Check sheet for the modelled part. Datum: model origin and axes. Units: mm. Face numbers are marked on the shaded views. A direction names the side the tool comes from. Coordinates: 2 decimals unless noted, no trailing zeros. Loops run counter-clockwise (first coordinate to the right, second up) from the corner with the lowest first, then second, coordinate; pieces in that order, holes last. Notation, with made-up numbers: M 35,24 L 76,24 A4 ccw 76,29 Z; hole C 50.25,78.5 d7. An arc over 180 degrees is marked long. Answer in a Markdown table with one row per item. Add a question column.
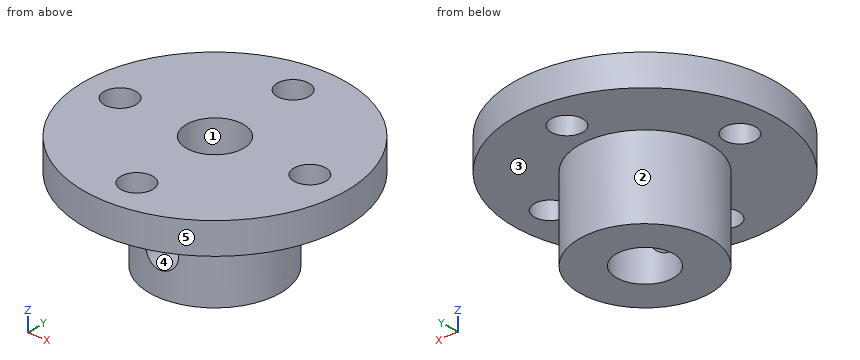
```python
from build123d import *

# Parameters (mm, degrees)
SKETCH1_R           = 8
SKETCH1_R_2         = 3.5
BOSS_EXTRUDE1_DEPTH = 10
SKETCH2_R           = 16
SKETCH2_R_2         = 3.5
BOSS_EXTRUDE2_DEPTH = 3.81
SKETCH3_R           = 1.95
CUT_EXTRUDE1_DEPTH  = 27.508792881
SKETCH4_R           = 2
CUT_EXTRUDE2_DEPTH  = 27.508792881


with BuildPart() as part:
    # Sketch1 → Boss-Extrude1 (new body)
    with BuildSketch(Plane.XY):
        Circle(SKETCH1_R)
        Circle(SKETCH1_R_2, mode=Mode.SUBTRACT)
    extrude(amount=BOSS_EXTRUDE1_DEPTH)

    # Sketch2 → Boss-Extrude2 (add)
    with BuildSketch(Plane.XY.offset(10)):
        with Locations(Location((0, 0, 0), (0, 0, 180))):
            Circle(SKETCH2_R)
        Circle(SKETCH2_R_2, mode=Mode.SUBTRACT)
    extrude(amount=BOSS_EXTRUDE2_DEPTH)

    # Sketch3 → Cut-Extrude1 (cut, through all)
    with BuildSketch(Plane.XY.offset(13.81)):
        with Locations((0, 11.43)):
            Circle(SKETCH3_R)
        with Locations((11.43, 0)):
            Circle(SKETCH3_R)
        with Locations((0, -11.43)):
            Circle(SKETCH3_R)
        with Locations((-11.43, 0)):
            Circle(SKETCH3_R)
    extrude(amount=-CUT_EXTRUDE1_DEPTH, mode=Mode.SUBTRACT)

    # Sketch4 → Cut-Extrude2 (cut, through all)
    with BuildSketch(Plane(origin=(0, 0, 0), x_dir=(1, 0, 0), z_dir=(0, 1, 0))):
        with Locations(Location((0, -5, 0), (0, 0, 270))):
            Circle(SKETCH4_R)
    extrude(amount=-CUT_EXTRUDE2_DEPTH, mode=Mode.SUBTRACT)


solid = part.part
```
Q1. Access from +Z, -Z, +X, -X, +Y, -Y to the whole of each face (thin tool, end or side, straight path). Record for the marked faces 1 and 2.
Q2. Thickness scan on L1, parallel to Y at x = 0, z = 11.25; L2, parallel to Y at x = 0, z = 8; L3, parallel to X at y = -4.5, z = 4.25. Record the ranges inside material, lowest first.
Q3. Cross-section at A-A (x = 0). Record the cut outline in (y, z).
Q4. Cross-section at B-B (y = -1). Record the cut outline in (x, z).
Q5. Cross-section at C-C (x = 11.43). Record the cut outline in (y, z), plus the area to 3 significant figures.
Q6. Cross-section at D-D (z = 13). Record the cut outline in (x, y), plus the area to 3 significant figures.
Q7. Mould release check, pull along X, two halves, no side actions. Record for the marked faces 3, 4 and 5: released by +X, released by -X, zero draft, split by the parting line, or undercut.
Q8. Go/stop test with flat-tipped pins: pin 1 (1.5 mm diameter, centred on y = -6.5, z = 10, fed in from +X); pin 2 (6 mm diameter, centred on x = 0, y = -11.43, fed in from -Z); pin 3 (2 mm diameter, centred on y = -5.5, z = 3, fed in from +X); pin 4 (3 mm diameter, centred on x = 0, y = 11.43, fed in from +Z). Record where each tip stops, or that it passes through.
Answer key:
| question | item | result |
|---|---|---|
| 1 | face 1 | +Z, -Z |
| 1 | face 2 | -Z |
| 2 | L1 | -16 to -13.38, -9.48 to -3.5, 3.5 to 9.48, 13.38 to 16 |
| 2 | L2 | -8 to -3.5, 3.5 to 8 |
| 2 | L3 | -6.61 to -1.85, 1.85 to 6.61 |
| 3 | outline | M -16,10 L -13.38,10 L -13.38,13.81 L -16,13.81 Z; M -9.48,10 L -8,10 L -8,7 L -3.5,7 L -3.5,13.81 L -9.48,13.81 Z; M -8,0 L -3.5,0 L -3.5,3 L -8,3 Z; M 3.5,0 L 8,0 L 8,10 L 9.48,10 L 9.48,13.81 L 3.5,13.81 Z; M 13.38,10 L 16,10 L 16,13.81 L 13.38,13.81 Z |
| 4 | outline | M -15.97,10 L -13.1,10 L -13.1,13.81 L -15.97,13.81 Z; M -9.76,10 L -7.94,10 L -7.94,0 L -3.35,0 L -3.35,13.81 L -9.76,13.81 Z; M 3.35,0 L 7.94,0 L 7.94,10 L 9.76,10 L 9.76,13.81 L 3.35,13.81 Z; M 13.1,10 L 15.97,10 L 15.97,13.81 L 13.1,13.81 Z |
| 5 | outline | M -11.2,10 L -1.95,10 L -1.95,13.81 L -11.2,13.81 Z; M 1.95,10 L 11.2,10 L 11.2,13.81 L 1.95,13.81 Z |
| 5 | area | 70.5 mm^2 |
| 6 | outline | C 0,0 d32; hole C -11.43,0 d3.9; hole C 0,0 d7; hole C 0,-11.43 d3.9; hole C 0,11.43 d3.9; hole C 11.43,0 d3.9 |
| 6 | area | 718 mm^2 |
| 7 | face 3 | zero draft |
| 7 | face 4 | undercut |
| 7 | face 5 | split by the parting line |
| 8 | pin 1 | x = 14.93 |
| 8 | pin 2 | z = 10 |
| 8 | pin 3 | x = 6.61 |
| 8 | pin 4 | through |
